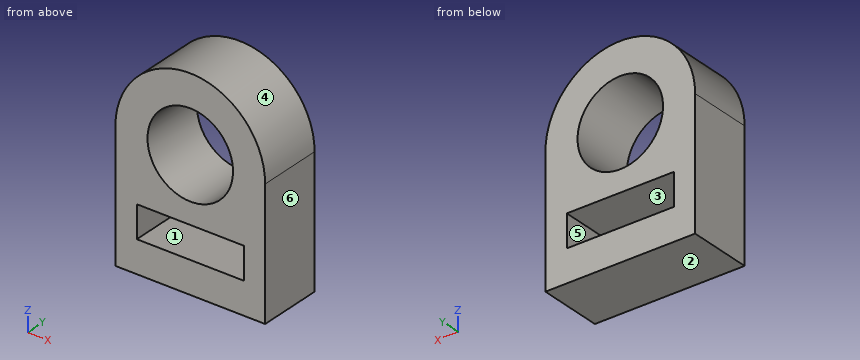
from build123d import *

# Parameters (mm, degrees)
F0_W     = 50
F0_H     = 15
F0_R     = 20
F1_DEPTH = 30


with BuildPart() as f1:
    # F0 (on Front) → F1 (new body)
    with BuildSketch(Plane.XZ):
        with BuildLine():
            Line((35, -60), (35, 0))
            ThreePointArc((35, 0), (0, 35), (-35, 0))
            Line((-35, 0), (-35, -60))
            Line((-35, -60), (35, -60))
        make_face()
        with Locations((0, -37.5)):
            Rectangle(F0_W, F0_H, mode=Mode.SUBTRACT)
        Circle(F0_R, mode=Mode.SUBTRACT)
    extrude(amount=F1_DEPTH)


solid = f1.part
Here's how the part is built. I have some questions about the finished solid (model axes, mm). Face numbers are marked on the shaded views. A direction names the side the tool comes from. Give positions to 0.01 mm unless a question says otherwise; leave off trailing zeros. Loops run counter-clockwise (first coordinate to the right, second up) from the corner with the lowest first, then second, coordinate; pieces in that order, holes last. Notation, with made-up numbers: (44, 84) -> (101, 84) arc R13 ccw to (101, 97) -> close; hole circle Ø10 at (-28, -35). An arc over 180 degrees is marked (long way). Answer as a JSON object with one key per item and string values. Group by question number.
Item 1: Thinking about a two-plate mould opening in Z: for the marked faces 3, 4, 5 and 6, which applies, pulls with the +Z half, pulls with the -Z half, needs draft (parallel to the pull), parting line crosses it, or undercut?
Item 2: Imagine slicing it at B-B on z = -16. Write out the boundary of the cut face in (x, y).
Item 3: I need wall thicknesses on L1, parallel to Z at x = 0, y = -22.75; L2, parallel to Z at x = 4.5, y = -22.75; L3, parallel to Z at x = 28, y = -11.5. Which ranges of each line are inside material? Lowest first, please.
Item 4: Imagine slicing it at D-D on y = -25.25. Write out the boundary of the cut face in (x, z), then the cut area to 3 significant figures.
Item 5: Will these pins go through, and if not, where does the flat tip stop? pin 1 (2 mm diameter, centred on y = -26.5, z = 3.5, fed in from -X); pin 2 (1.5 mm diameter, centred on x = 17, y = -24, fed in from +Z); pin 3 (2 mm diameter, centred on x = 21.5, y = -18, fed in from +Z); pin 4 (5 mm diameter, centred on x = 9.5, z = 14, fed in from -Y).
Item 6: On a 3-axis mill with a long thin cutter (end or side, diameter ignored), from which of +Z, -Z, +X, -X, +Y, -Y can I reach the whole of each face in a straight line? I mean the marked faces 1 and 2. Say none if no direction works.
Item 7: Imagine slicing it at A-A on x = 21. Write out the boundary of the cut face in (y, z).
Item 8: Imagine slicing it at C-C on x = 0. Write out the boundary of the cut face in (y, z), then the cut area to 3 significant figures.
Answer list:
{
 "1": {"face 3": "undercut", "face 4": "pulls with the +Z half", "face 5": "undercut", "face 6": "needs draft"},
 "2": {"outline": "(-35, -30) -> (-12, -30) -> (-12, 0) -> (-35, 0) -> close; (12, -30) -> (35, -30) -> (35, 0) -> (12, 0) -> close"},
 "3": {"L1": "z = -60 to -45, -30 to -20, 20 to 35", "L2": "z = -60 to -45, -30 to -19.49, 19.49 to 34.71", "L3": "z = -60 to 21"},
 "4": {"outline": "(-35, -60) -> (35, -60) -> (35, 0) arc R35 ccw to (-35, 0) -> close; hole (-25, -45) -> (25, -45) -> (25, -30) -> (-25, -30) -> close; hole circle Ø40 at (0, 0)", "area": "4,120 mm2"},
 "5": {"pin 1": "stops at x = -34.91", "pin 2": "stops at z = 31", "pin 3": "stops at z = 28.37", "pin 4": "passes through"},
 "6": {"face 1": "+Y, -Y", "face 2": "-Z, +X, -X, +Y, -Y"},
 "7": {"outline": "(-30, -60) -> (0, -60) -> (0, -45) -> (-30, -45) -> close; (-30, -30) -> (0, -30) -> (0, 28) -> (-30, 28) -> close"},
 "8": {"outline": "(-30, -60) -> (0, -60) -> (0, -45) -> (-30, -45) -> close; (-30, -30) -> (0, -30) -> (0, -20) -> (-30, -20) -> close; (-30, 20) -> (0, 20) -> (0, 35) -> (-30, 35) -> close", "area": "1,200 mm2"}
}
